Check sheet for the modelled part. Datum: model origin and axes. Units: mm. Coordinates: 2 decimals unless noted, no trailing zeros. Write each loop counter-clockwise with the first axis right and the second up, starting at its lowest first coordinate (ties: lowest second). Pieces come first, ordered by that corner, then holes. Notation, with made-up numbers: (-38, 84) -> (14, 84) arc R15 cw to (14, 112) -> close; hole circle Ø10 at (37.25, 60). An arc over 180 degrees is marked (long way). One line per item, written item: value. Start each with the question number.
1) Sectioned sample at A-A on z = 0. Enter the section's corners in (x, y), plus the area to 3 significant figures.
2) Gauge pin test, flat end, axial feed: P1, Ø1, axis at x = 37, y = 1.5, coming from the +Z side. Record the tip position at first contact, or that the pin passes through.
3) Sectioned sample at C-C on y = 1.1. Enter the section's corners in (x, z).
4) Scan lines: line 1 along X through (y, z) = (1.35, 0); line 2 along Z through (x, y) = (-1.5, 0.8); line 3 along Z through (x, y) = (25.5, 0.55). Record each from-to range of solid material in increasing order. Write a range as [from, to].
5) Draft check along X on faces 1 (the flat face through (-41, 2, -37)), 2 (the cylindrical face through (-45.65, 0.99, -46.27)), 3 (the cylindrical face through (-48.794, 0.986, 25.379)). Enter one of: +X half, -X half, draft (parallel to the pull), parting line (faces both ways), or undercut.
6) Sectioned sample at B-B on x = 0. Enter the section's corners in (y, z).
```python
from build123d import *

# Parameters (mm, degrees)
SKETCH_1_R          = 65
SKETCH_1_R_2        = 55
EXTRUDE_1_DEPTH     = 2
SKETCH_3_W          = 168.977595328
SKETCH_3_H          = 144.759308048
SKETCH_3_W_2        = 124
SKETCH_3_H_2        = 124
CUT_EXTRUDE_1_DEPTH = 3
SKETCH_4_R          = 1.25
CUT_EXTRUDE_2_DEPTH = 3


with BuildPart() as part:
    # 草图1 → 凸台-拉伸1 (new body)
    with BuildSketch(Plane(origin=(0, 0, 0), x_dir=(1, 0, 0), z_dir=(0, 1, 0))):
        with Locations(Location((0, 0, 0), (0, 0, 270))):
            Circle(SKETCH_1_R)
        with Locations(Location((0, 0, 0), (0, 0, 270))):
            Circle(SKETCH_1_R_2, mode=Mode.SUBTRACT)
    extrude(amount=EXTRUDE_1_DEPTH)

    # 草图3 → 切除-拉伸1 (cut)
    with BuildSketch(Plane(origin=(0, 2, 0), x_dir=(1, 0, 0), z_dir=(0, 1, 0))):
        Rectangle(SKETCH_3_W, SKETCH_3_H)
        Rectangle(SKETCH_3_W_2, SKETCH_3_H_2, mode=Mode.SUBTRACT)
    extrude(amount=-CUT_EXTRUDE_1_DEPTH, mode=Mode.SUBTRACT)

    # 草图4 → 切除-拉伸2 (cut)
    with BuildSketch(Plane(origin=(0, 2, 0), x_dir=(1, 0, 0), z_dir=(0, 1, 0))):
        with Locations(Location((43.133513652, -43.133513652, 0), (0, 0, 270))):
            Circle(SKETCH_4_R)
        with Locations(Location((-43.133513652, -43.133513652, 0), (0, 0, 270))):
            Circle(SKETCH_4_R)
        with Locations(Location((-43.133513652, 43.133513652, 0), (0, 0, 270))):
            Circle(SKETCH_4_R)
        with Locations(Location((43.133513652, 43.133513652, 0), (0, 0, 270))):
            Circle(SKETCH_4_R)
    extrude(amount=-CUT_EXTRUDE_2_DEPTH, mode=Mode.SUBTRACT)


solid = part.part
```
Answers:
1. outline: (-62, 0) -> (-55, 0) -> (-55, 2) -> (-62, 2) -> close; (55, 0) -> (62, 0) -> (62, 2) -> (55, 2) -> close
1. area: 28.0 mm2
2. P1: stops at z = 53.78
3. outline: (-62, -19.52) arc R65 ccw to (-19.52, -62) -> (19.52, -62) arc R65 ccw to (62, -19.52) -> (62, 19.52) arc R65 ccw to (19.52, 62) -> (-19.52, 62) arc R65 ccw to (-62, 19.52) -> close; hole circle Ø110 at (0, 0); hole circle Ø2.5 at (-43.13, -43.13); hole circle Ø2.5 at (-43.13, 43.13); hole circle Ø2.5 at (43.13, -43.13); hole circle Ø2.5 at (43.13, 43.13)
4. line 1: x = [-62, -55], [55, 62]
4. line 2: z = [-62, -54.98], [54.98, 62]
4. line 3: z = [-59.79, -48.73], [48.73, 59.79]
5. face 1: draft
5. face 2: -X half
5. face 3: undercut
6. outline: (0, -62) -> (2, -62) -> (2, -55) -> (0, -55) -> close; (0, 55) -> (2, 55) -> (2, 62) -> (0, 62) -> close
